Check sheet for the modelled part. Datum: model origin and axes. Units: mm. A direction names the side the tool comes from. Give positions to 0.01 mm unless a question says otherwise; leave off trailing zeros. Loops run counter-clockwise (first coordinate to the right, second up) from the corner with the lowest first, then second, coordinate; pieces in that order, holes last. Notation, with made-up numbers: (64, 42.5) - (118, 42.5) arc R29 cw to (118, 81.5) - close; hole circle Ø5 at (44.5, 26). An arc over 180 degrees is marked (long way). Answer in a Markdown table with one row per item. Add a question column.
(1) Set-up check for faces 1 (the face through (67, 39, 0)), 2 (the face through (90, 70, 6)): record each of +Z, -Z, +X, -X, +Y, -Y from which the full face is reachable in a straight line by a thin tool's end or side.
(2) Sectioned sample at C-C on x = 90. Enter the section's corners in (y, z), then the cut area to 3 significant figures.
(3) Sectioned sample at A-A on x = 7.5. Enter the section's corners in (y, z).
(4) Thickness scan on L1, parallel to Y at x = 7.5, z = 2.5; L2, parallel to Y at x = 75, z = 8.7; L3, parallel to Y at x = 90, z = 2.4. Record the ranges inside material, lowest first.
(5) Sectioned sample at D-D on y = 10.4. Enter the section's corners in (x, z).
(6) Go/stop test with flat-tipped pins: P1, Ø6.5, axis at x = 7.5, y = 67.4, coming from the +Z side; P2, Ø3, axis at x = 90, y = 71.5, coming from the +Z side; P3, Ø5, axis at x = 7.5, y = 10.4, coming from the -Z side. Record where each tip stops, or that it passes through.
(7) Draft check along Y on faces 3 (the face through (123.36, 44.1, 8.03)), 4 (the face through (0, 38, 5)), 5 (the face through (67, 77.4, 5)). Enter one of: released by +Y, released by -Y, zero draft, split by the parting line, or undercut.
(8) Sectioned sample at B-B on y = 43.2. Enter the section's corners in (x, z), then the cut area to 3 significant figures.
from build123d import *

# Parameters (mm, degrees)
SKETCH_1_W                   = 135.5
SKETCH_1_H                   = 77.4
EXTRUDE_1_DEPTH              = 10
HOLE_WIZARD_M3_1_D           = 3.4
HOLE_WIZARD_M3_1_CBORE_D     = 6
HOLE_WIZARD_M3_1_CBORE_DEPTH = 4
HOLE_WIZARD_M3_2_D           = 3.4
HOLE_WIZARD_M3_2_CBORE_D     = 6
HOLE_WIZARD_M3_2_CBORE_DEPTH = 4
HOLE_WIZARD_M5_1_D           = 5.5
HOLE_WIZARD_M5_1_CBORE_D     = 10
HOLE_WIZARD_M5_1_CBORE_DEPTH = 6


with BuildPart() as part:
    # ｽｹｯﾁ1 → ﾎﾞｽ - 押し出し1 (new body)
    with BuildSketch(Plane.XY):
        with Locations((67.75, 38.7)):
            Rectangle(SKETCH_1_W, SKETCH_1_H)
    extrude(amount=EXTRUDE_1_DEPTH)

    # M3 穴付きねじ用座ぐり穴1 (through all)
    with Locations(Plane.XY.offset(10)):
        with Locations((130.5, 43.2), (120.5, 43.2)):
            CounterBoreHole(HOLE_WIZARD_M3_1_D / 2, HOLE_WIZARD_M3_1_CBORE_D / 2, HOLE_WIZARD_M3_1_CBORE_DEPTH)

    # M3 穴付きねじ用座ぐり穴2 (through all)
    with Locations(Plane.XY.offset(10)):
        with Locations((130.5, 43.2), (75, 72.4), (90, 72.4), (120.5, 43.2)):
            CounterBoreHole(HOLE_WIZARD_M3_2_D / 2, HOLE_WIZARD_M3_2_CBORE_D / 2, HOLE_WIZARD_M3_2_CBORE_DEPTH)

    # M5 穴付きねじ用座ぐり穴1 (through all)
    with Locations(Plane.XY.offset(10)):
        with Locations((7.5, 67.4), (7.5, 10.4)):
            CounterBoreHole(HOLE_WIZARD_M5_1_D / 2, HOLE_WIZARD_M5_1_CBORE_D / 2, HOLE_WIZARD_M5_1_CBORE_DEPTH)


solid = part.part
Reply:
| question | item | result |
|---|---|---|
| 1 | face 1 | -Z, +X, -X, +Y, -Y |
| 1 | face 2 | +Z |
| 2 | outline | (0, 0) - (70.7, 0) - (70.7, 6) - (69.4, 6) - (69.4, 10) - (0, 10) - close; (74.1, 0) - (77.4, 0) - (77.4, 10) - (75.4, 10) - (75.4, 6) - (74.1, 6) - close |
| 2 | area | 730 mm^2 |
| 3 | outline | (0, 0) - (7.65, 0) - (7.65, 4) - (5.4, 4) - (5.4, 10) - (0, 10) - close; (13.15, 0) - (64.65, 0) - (64.65, 4) - (62.4, 4) - (62.4, 10) - (15.4, 10) - (15.4, 4) - (13.15, 4) - close; (70.15, 0) - (77.4, 0) - (77.4, 10) - (72.4, 10) - (72.4, 4) - (70.15, 4) - close |
| 4 | L1 | 0 to 7.65, 13.15 to 64.65, 70.15 to 77.4 |
| 4 | L2 | 0 to 69.4, 75.4 to 77.4 |
| 4 | L3 | 0 to 70.7, 74.1 to 77.4 |
| 5 | outline | (0, 0) - (4.75, 0) - (4.75, 4) - (2.5, 4) - (2.5, 10) - (0, 10) - close; (10.25, 0) - (135.5, 0) - (135.5, 10) - (12.5, 10) - (12.5, 4) - (10.25, 4) - close |
| 6 | P1 | z = 4 |
| 6 | P2 | z = 6 |
| 6 | P3 | through |
| 7 | face 3 | undercut |
| 7 | face 4 | zero draft |
| 7 | face 5 | released by +Y |
| 8 | outline | (0, 0) - (118.8, 0) - (118.8, 6) - (117.5, 6) - (117.5, 10) - (0, 10) - close; (122.2, 0) - (128.8, 0) - (128.8, 6) - (127.5, 6) - (127.5, 10) - (123.5, 10) - (123.5, 6) - (122.2, 6) - close; (132.2, 0) - (135.5, 0) - (135.5, 10) - (133.5, 10) - (133.5, 6) - (132.2, 6) - close |
| 8 | area | 1,270 mm^2 |
